Autodesk Inventor part; units mm, degrees
ref_plane "YZ Plane" through (0, 0, 0) normal (1, 0, 0) x (0, 1, 0)
ref_plane "XZ Plane" through (0, 0, 0) normal (0, 1, 0) x (-1, 0, 0)
ref_plane "XY Plane" through (0, 0, 0) normal (0, 0, 1) x (1, 0, 0)
sketch "Sketch1" plane through (0, 0, 0) normal (0, 0, 1) x (1, 0, 0)
  line L0 (0, 0) -> (152.4, 0)
  line L1 (152.4, 0) -> (152.4, 152.4)
  line L2 (0, 152.4) -> (0, 0)
  line L3 (88.9, 152.4) -> (88.9, 165.1)
  line L4 (88.9, 165.1) -> (76.2, 165.1)
  line L5 (76.2, 165.1) -> (63.5, 165.1)
  line L6 (63.5, 165.1) -> (63.5, 152.4)
  line L7 (152.4, 152.4) -> (88.9, 152.4)
  line L8 (63.5, 152.4) -> (0, 152.4)
  circle A0 centre (38.1, 114.3) radius 12.7
  circle A1 centre (114.3, 114.3) radius 12.7
  circle A2 centre (76.2, 76.2) radius 12.7
  circle A3 centre (38.1, 38.1) radius 12.7
  circle A4 centre (114.3, 38.1) radius 12.7
  line L9 (63.5, 152.4) -> (63.5, -12.7)
  line L10 (88.9, 152.4) -> (88.9, -12.7)
  line L11 (63.5, 0) -> (88.9, 0)
  line L12 (88.9, 0) -> (88.9, -12.7)
  line L13 (88.9, -12.7) -> (63.5, -12.7)
  line L14 (63.5, -12.7) -> (63.5, 0)
  dimension "d0" = 152.4
  dimension "d1" = 152.4
  dimension "d5" = 12.7
  dimension "d6" = 12.7
  dimension "d7" = 12.7
  dimension "d8" = 12.7
  dimension "d9" = 63.5
  dimension "d10" = 90
  dimension "d11" = 25.4
  dimension "d12" = 25.4
  dimension "d13" = 25.4
  dimension "d14" = 25.4
  dimension "d15" = 25.4
  dimension "d16" = 38.1
  dimension "d17" = 38.1
  dimension "d18" = 38.1
  dimension "d19" = 38.1
  dimension "d20" = 76.2
  dimension "d21" = 76.2
  dimension "d22" = 38.1
  dimension "d23" = 38.1
  dimension "d24" = 38.1
  dimension "d25" = 38.1
  dimension "d26" = 12.7
extrude "Extrusion1" add sketch "Sketch1" along normal blind 5.08 contours L2 L8 L9 L0 | L9 A2 L10 L0 | L0 L10 L13 L9 | L10 L7 L1 L0 | L9 L6 L5 L4 L3 L10 A2
sketch "Sketch2" plane through (0, 0, 0) normal (0, -1, 0) x (1, 0, 0)
  line L0 (63.5, 5.08) -> (0, 5.08)
  line L1 (0, 0) -> (12.7, 0)
  line L2 (12.7, 0) -> (12.7, 5.08)
  line L3 (12.7, 5.08) -> (0, 5.08)
  line L4 (0, 5.08) -> (0, 0)
  line L5 (88.9, 5.08) -> (152.4, 5.08)
  line L6 (152.4, 0) -> (139.7, 0)
  line L7 (139.7, 0) -> (139.7, 5.08)
  line L8 (139.7, 5.08) -> (152.4, 5.08)
  line L9 (152.4, 5.08) -> (152.4, 0)
  dimension "d29" = 12.7
  dimension "d31" = 12.7
extrude "Extrusion2" add sketch "Sketch2" along normal blind 12.7
properties part number "Heating Plate"
Geometry: final body of the model. Coordinates: model frame, mm. A direction names the side the tool comes from. Round coordinates to 2 decimals unless told otherwise and drop trailing zeros. Write each loop counter-clockwise with the first axis right and the second up, starting at its lowest first coordinate (ties: lowest second). Pieces come first, ordered by that corner, then holes.
Item 1: Material intervals for L1, parallel to Y at x = 38.1, z = 2.9; L2, parallel to X at y = 76.2, z = 3.35, sorted ascending.
Item 2: Section query B-B (x = 114.3). Return loops of the section in (y, z).
Item 3: Section query C-C (z = 1.4). Return loops of the section in (x, y), plus the area to 3 significant figures.
Item 4: Section query A-A (y = 76.2). Return loops of the section in (x, z).
Item 5: Mould query, pull axis Y, two halves, no side actions, for faces 1 (the face through (101.612, 113.742, 2.504)), 2 (the face through (6, -12.7, 3)), 3 (the face through (58, 77, 0)), 4 (the face through (49.832, 42.964, 2.504)). Classes: +Y half, -Y half, draft (parallel to the pull), parting line (faces both ways), or undercut.
Item 6: Pin query (flat end, axial travel): P1, Ø2.5, axis at x = 39.5, z = 2, coming from the -Y side; P2, Ø1.5, axis at y = 161.5, z = 3, coming from the +X side. Return the tip coordinate at first contact, or that it passes through.
Item 7: Set-up query: faces 5 (the face through (88.9, 159, 3)), 6 (the face through (32, 152.4, 3)), 7 (the face through (114, 0, 3)), 8 (the face through (0, 71, 3)), 9 (the face through (146, -12.7, 3)). Return all of +Z, -Z, +X, -X, +Y, -Y with unobstructed straight access to the full face (end or side cutting, diameter ignored); none if empty.
Completed:
1. L1: y = 0 to 25.4, 50.8 to 101.6, 127 to 152.4
1. L2: x = 0 to 63.5, 88.9 to 152.4
2. outline: (0, 0) - (25.4, 0) - (25.4, 5.08) - (0, 5.08) - close; (50.8, 0) - (101.6, 0) - (101.6, 5.08) - (50.8, 5.08) - close; (127, 0) - (152.4, 0) - (152.4, 5.08) - (127, 5.08) - close
3. outline: (0, -12.7) - (12.7, -12.7) - (12.7, 0) - (63.5, 0) - (63.5, -12.7) - (88.9, -12.7) - (88.9, 0) - (139.7, 0) - (139.7, -12.7) - (152.4, -12.7) - (152.4, 152.4) - (88.9, 152.4) - (88.9, 165.1) - (63.5, 165.1) - (63.5, 152.4) - (0, 152.4) - close; hole circle Ø25.4 at (38.1, 38.1); hole circle Ø25.4 at (38.1, 114.3); hole circle Ø25.4 at (76.2, 76.2); hole circle Ø25.4 at (114.3, 38.1); hole circle Ø25.4 at (114.3, 114.3)
3. area: 21,700 mm2
4. outline: (0, 0) - (63.5, 0) - (63.5, 5.08) - (0, 5.08) - close; (88.9, 0) - (152.4, 0) - (152.4, 5.08) - (88.9, 5.08) - close
5. face 1: undercut
5. face 2: -Y half
5. face 3: draft
5. face 4: undercut
6. P1: stops at y = 0
6. P2: stops at x = 88.9
7. face 5: +Z, -Z, +X, +Y
7. face 6: +Z, -Z, -X, +Y
7. face 7: +Z, -Z, -Y
7. face 8: +Z, -Z, -X, +Y, -Y
7. face 9: +Z, -Z, +X, -X, -Y
